```python
from build123d import *


with BuildPart() as part:
    # Sketch → Revolution (revolve)
    with BuildSketch(Plane.YZ):
        Polygon((250, 0), (250, 25), (5, 25), (5, 80), (0, 80), (0, 0), align=None)
    revolution = revolve(axis=Axis((0, 0, 0), (0, 0, 1)))

    # Mirrored: Revolution across Sketch H_Axis
    add(revolution.mirror(Plane.XY))


solid = part.part
```
Model file for the job. Use its own axes, mm. Round coordinates to 2 decimals unless told otherwise and drop trailing zeros. Loops run counter-clockwise (first coordinate to the right, second up) from the corner with the lowest first, then second, coordinate; pieces in that order, holes last. Notation, with made-up numbers: M 5.25,-8 L 40.25,-8 A15 ccw 40.25,6 Z; hole C -2.75,13.5 d10. An arc over 180 degrees is marked long. Put each result on its own line as item: value. Start each with the question number.
Item 1: Cut at B-B (x = 161.5). List the corners of the cut face in (y, z).
Item 2: Drop flat-ended pins along their axis: P1, Ø10, axis at y = -3.5, z = 55.5, coming from the -X side; P2, Ø5, axis at x = 135, z = 6, coming from the -Y side; P3, Ø1.5, axis at x = -13.5, y = -160.5, coming from the +Z side; P4, Ø8, axis at x = 68, z = -30, coming from the +Y side. Give the stop position or say it passes through.
Item 3: Cut at C-C (y = -52.5). List the corners of the cut face in (x, z).
Item 4: Drill centre lines: line 1 along Z through (x, y) = (134, -178); line 2 along Y through (x, z) = (-0.5, -21); line 3 along Y through (x, z) = (56, -7). Where is each one in solid material? Low to high.
Item 5: Cut at A-A (z = -47). List the corners of the cut face in (x, y).
Answer block:
1. outline: M -190.83,-25 L 190.83,-25 L 190.83,25 L -190.83,25 Z
2. P1: x = -5
2. P2: y = -212
2. P3: z = 25
2. P4: through
3. outline: M -244.43,-25 L 244.43,-25 L 244.43,25 L -244.43,25 Z
4. line 1: -25 to 25
4. line 2: -250 to 250
4. line 3: -243.65 to 243.65
5. outline: C 0,0 d10
